The listing builds one solid part. Answer for the finished solid, in the listing's coordinates (mm). Round coordinates to 2 decimals unless told otherwise and drop trailing zeros. Order: outer loops, then holes, each group sorted by start corner. A loop starts at its lowest first (then second) coordinate and runs counter-clockwise, first axis right, second up. Notation, with made-up numbers: M 63,70 L 90,70 A10 ccw 90,85 Z; hole C 35,-13 d10. An arc over 180 degrees is marked long. Write item = value, one per line. Start each with the question number.
(1) Each of these flat-tipped pins is pushed along its axis until it touches: pin 1 (7 mm diameter, centred on x = 35, y = 0, fed in from -Z); pin 2 (6.5 mm diameter, centred on x = -28.28, y = 28.28, fed in from -Z); pin 3 (3 mm diameter, centred on y = -12, z = 5, fed in from +X); pin 4 (1 mm diameter, centred on y = 19, z = 2, fed in from +X). Where does it stop, or does it pass through?
(2) A cutting plane is placed at C-C, the plane z = 4. Determine the outline of the cut face in (x, y), and give its area (3 significant figures).
(3) Straight lines are drawn through the part: probe 1 along Y at (x, z) = (0, 4.5); probe 2 along X at (y, z) = (-13.5, 1); probe 3 along Y at (x, z) = (15.5, 7.25). For each, find the intervals that lie inside material, in ascending order. Write a range as from..to.
(4) For a pull along X with two mould halves and no side action, classify faces 1 (the face through (-22.9, -10.4, 0)), 2 (the face through (-27.62, 30.4, 1.78)), 3 (the face through (26.42, -29.25, 4.99)), 4 (the face through (47.69, -15.02, 3.94)) as released by +X, released by -X, zero draft, split by the parting line, or undercut.
(5) A cutting plane is placed at A-A, the plane x = 0. Determine the outline of the cut face in (y, z), and give its area (3 significant figures).
(6) A cutting plane is placed at D-D, the plane y = -35. Determine the outline of the cut face in (x, z).
Autodesk Inventor part; units mm, degrees
ref_plane "YZ Plane" through (0, 0, 0) normal (1, 0, 0) x (0, 1, 0)
ref_plane "XZ Plane" through (0, 0, 0) normal (0, 1, 0) x (-1, 0, 0)
ref_plane "XY Plane" through (0, 0, 0) normal (0, 0, 1) x (1, 0, 0)
sketch "Sketch2" plane through (0, 0, 0) normal (0, 0, 1) x (1, 0, 0)
  circle A0 centre (0, 0) radius 25
  circle A1 centre (0, 0) radius 50
  dimension "d11" = 100
  dimension "d12" = 50
extrude "Extrusion2" add sketch "Sketch2" along normal blind 8
sketch "Sketch3" plane through (0, 0, 8) normal (0, 0, 1) x (1, 0, 0)
  point P0 (0, 0)
  point P1 (35, 0)
  dimension "d15" = 35
hole "Hole1" at (35, 0, 8) direction (0, 0, -1) diameter 4.5 depth 8 tip angle 118
pattern_circular "Circular Pattern1" count 4 over 360 about axis through (0, 0, 0) along (0, 0, 1) of "Hole1"
sketch "Sketch4" plane through (0, 0, 0) normal (0, 0, -1) x (-1, 0, 0)
  line L0 (0, 0) -> (28.2843, 28.2843)
  line L1 (0, 0) -> (17.6035, 0)
  dimension "d26" = 45
  dimension "d27" = 40
hole "Hole2" at (-28.2843, 28.2843, 0) direction (0, 0, 1) diameter 4.2 depth 8 tip angle 118 countersink diameter 8 countersink angle 90
pattern_circular "Circular Pattern2" count 2 over 360 about axis through (0, 0, 0) along (0, 0, 1) of "Hole2"
properties part number "M20 - Flange Connector" material "ABS Plastic"
Reported:
q1.pin_1 = 0
q1.pin_2 = 0.74
q1.pin_3 = 48.89
q1.pin_4 = 46.45
q2.outline = C 0,0 d100; hole C -35,0 d4.5; hole C -28.28,28.28 d4.2; hole C 0,0 d50; hole C 0,-35 d4.5; hole C 0,35 d4.5; hole C 28.28,-28.28 d4.2; hole C 35,0 d4.5
q2.area = 5,800 mm²
q3.probe_1 = -50..-37.25, -32.75..-25, 25..32.75, 37.25..50
q3.probe_2 = -48.14..-21.04, 21.04..48.14
q3.probe_3 = -47.54..-19.62, 19.62..47.54
q4.face_1 = zero draft
q4.face_2 = undercut
q4.face_3 = undercut
q4.face_4 = split by the parting line
q5.outline = M -50,0 L -37.25,0 L -37.25,8 L -50,8 Z; M -32.75,0 L -25,0 L -25,8 L -32.75,8 Z; M 25,0 L 32.75,0 L 32.75,8 L 25,8 Z; M 37.25,0 L 50,0 L 50,8 L 37.25,8 Z
q5.area = 328 mm²
q6.outline = M -35.71,0 L -2.25,0 L -2.25,8 L -35.71,8 Z; M 2.25,0 L 35.71,0 L 35.71,8 L 2.25,8 Z
